For this review, take the finished solid that the model builds, in its own axes (mm). A direction names the side the tool comes from. Give positions to 0.01 mm unless a question says otherwise; leave off trailing zeros. Loops run counter-clockwise (first coordinate to the right, second up) from the corner with the lowest first, then second, coordinate; pieces in that order, holes last. Notation, with made-up numbers: (60.5, -16) - (73.5, -16) arc R7 ccw to (73.5, -5) - close; hole circle Ø8 at (24, -33). An arc over 180 degrees is marked (long way). Use CSV: the item, a comma, the result in double quotes. Start each with the question number.
1. Take a section at C-C on z = 3.5. Give the boundary of the cut face in (x, y), plus the area to 3 significant figures.
2. Mouldability with a two-part tool opening along X and no side actions: class faces 1 (the flat face through (3, 0, 9.2)), 2 (the cylindrical face through (-9.97, -11.57, 0.61)), 3 (the flat face through (-1.424, 0, 5)), 4 (the cylindrical face through (11.38, 12, 0.61)) as pulls with the +X half, pulls with the -X half, needs draft (parallel to the pull), parting line crosses it, or undercut.
3. For faces 5 (the cylindrical face through (3.03, 9.13, 0.61)), 6 (the flat face through (3, -5.6, 5)), 7 (the flat face through (3, 5.6, 5)), 8 (the flat face through (7.95, 0, 5)), 9 (the cylindrical face through (11.35, -12.03, 0.61)), list the 3-axis set-ups (+Z, -Z, +X, -X, +Y, -Y) from which the entire face can be reached by the end or side of a thin tool; tool diameter is ignored.
4. Take a section at B-B on y = -2.5. Give the boundary of the cut face in (x, z).
5. Take a section at D-D on x = -3. Give the boundary of the cut face in (y, z), plus the area to 3 significant figures.
6. Wall thickness on line 1 (Y direction, x = -9.7, z = 0.7); line 2 (X direction, y = -4.75, z = 8.5); line 3 (Z direction, x = 11, y = 2.5): over which ranges is each line inside the solid? List them lowest first.
7. Take a section at A-A on x = 3.3. Give the boundary of the cut face in (y, z), plus the area to 3 significant figures.
8. For pin 1 (2.5 mm diameter, centred on y = -1.5, z = 3.5, fed in from +X); pin 2 (10 mm diameter, centred on x = -8.5, y = 7.5, fed in from +Z); pin 3 (3 mm diameter, centred on x = -9.7, y = 10.35, fed in from -Z); pin 4 (1.5 mm diameter, centred on x = 3.3, y = -10.35, fed in from +Z), all flat-tipped, find the tip position at first contact; note any pin that passes through.
```python
from build123d import *

# Parameters (mm, degrees)
CROQUIS1_W              = 25.2
CROQUIS1_H              = 23.9
SALIENTE_EXTRUIR1_DEPTH = 1.2
CROQUIS2_R              = 1.25
CORTAR_EXTRUIR1_DEPTH   = 1.2
REDONDEO1_R             = 2
CROQUIS3_W              = 9.37393079
CROQUIS3_H              = 11.2
SALIENTE_EXTRUIR2_DEPTH = 8


with BuildPart() as part:
    # Croquis1 → Saliente-Extruir1 (new body)
    with BuildSketch(Plane(origin=(0, 0, 0), x_dir=(0, 1, 0), z_dir=(0, 0, 1))):
        Rectangle(CROQUIS1_W, CROQUIS1_H)
    extrude(amount=SALIENTE_EXTRUIR1_DEPTH)

    # Croquis2 → Cortar-Extruir1 (cut)
    with BuildSketch(Plane.XY.offset(1.2)):
        with Locations((-9.7, -10.35)):
            Circle(CROQUIS2_R)
        with Locations((3.3, -10.35)):
            Circle(CROQUIS2_R)
        with Locations((3.3, 10.35)):
            Circle(CROQUIS2_R)
        with Locations((-9.7, 10.35)):
            Circle(CROQUIS2_R)
    extrude(amount=-CORTAR_EXTRUIR1_DEPTH, mode=Mode.SUBTRACT)

    # Redondeo1
    redondeo1_edges = [part.edges().sort_by_distance(p)[0] for p in [
        (11.95, 12.6, 0.6),
        (11.95, -12.6, 0.6),
        (-11.95, -12.6, 0.6),
        (-11.95, 12.6, 0.6),
    ]]
    fillet(redondeo1_edges, radius=REDONDEO1_R)

    # Croquis3 → Saliente-Extruir2 (add)
    with BuildSketch(Plane.XY.offset(1.2)):
        with Locations((3.263034605, 0)):
            Rectangle(CROQUIS3_W, CROQUIS3_H)
    extrude(amount=SALIENTE_EXTRUIR2_DEPTH)


solid = part.part
```
Check result:
1,outline,"(-1.42, -5.6) - (7.95, -5.6) - (7.95, 5.6) - (-1.42, 5.6) - close"
1,area,"105 mm²"
2,face 1,"needs draft"
2,face 2,"undercut"
2,face 3,"pulls with the -X half"
2,face 4,"pulls with the +X half"
3,face 5,"+Z, -Z"
3,face 6,"+Z, +X, -X, -Y"
3,face 7,"+Z, +X, -X, +Y"
3,face 8,"+Z, +X, +Y, -Y"
3,face 9,"+Z, -Z, +X, -Y"
4,outline,"(-11.95, 0) - (11.95, 0) - (11.95, 1.2) - (7.95, 1.2) - (7.95, 9.2) - (-1.42, 9.2) - (-1.42, 1.2) - (-11.95, 1.2) - close"
5,outline,"(-12.6, 0) - (12.6, 0) - (12.6, 1.2) - (-12.6, 1.2) - close"
5,area,"30.2 mm²"
6,line 1,"y = -12.6 to -11.6, -9.1 to 9.1, 11.6 to 12.6"
6,line 2,"x = -1.42 to 7.95"
6,line 3,"z = 0 to 1.2"
7,outline,"(-12.6, 0) - (-11.6, 0) - (-11.6, 1.2) - (-12.6, 1.2) - close; (-9.1, 0) - (9.1, 0) - (9.1, 1.2) - (5.6, 1.2) - (5.6, 9.2) - (-5.6, 9.2) - (-5.6, 1.2) - (-9.1, 1.2) - close; (11.6, 0) - (12.6, 0) - (12.6, 1.2) - (11.6, 1.2) - close"
7,area,"114 mm²"
8,pin 1,"stops at x = 7.95"
8,pin 2,"stops at z = 1.2"
8,pin 3,"stops at z = 0"
8,pin 4,"passes through"
